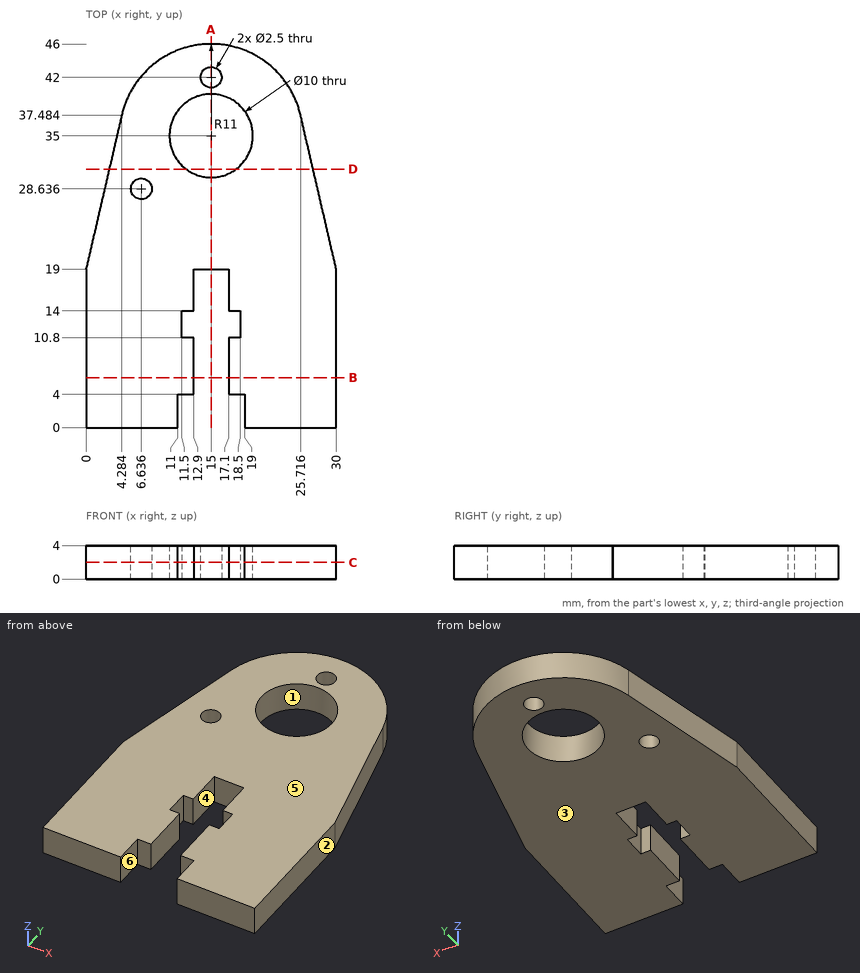
Geometry: see drawing. Coordinates: mm, zero at the bounding-box minimum. A direction names the side the tool comes from. Give positions to 0.01 mm unless a question says otherwise; leave off trailing zeros. Order: outer loops, then holes, each group sorted by start corner. A loop starts at its lowest first (then second) coordinate and runs counter-clockwise, first axis right, second up.
1. Cut plane A-A (x = 15). Return loops of the section in (y, z), and give its area (3 significant figures).
Computed:
outline: (19, 0) - (30, 0) - (30, 4) - (19, 4) - close; (40, 0) - (40.75, 0) - (40.75, 4) - (40, 4) - close; (43.25, 0) - (46, 0) - (46, 4) - (43.25, 4) - close
area: 58.0 mm2
2. Set-up query: the marked faces 5 and 6. Return all of +Z, -Z, +X, -X, +Y, -Y with unobstructed straight access to the full face (end or side cutting, diameter ignored); none if empty.
Computed:
face 5: +Z, +X, -X, +Y, -Y
face 6: +Z, -Z, -Y
3. Pin query (flat end, axial travel): pin 1 Ø1.2 at (x, z) = (15, 2.5) entering from -Y; pin 2 Ø0.7 at (x, z) = (12.5, 1.5) entering from -Y; pin 3 Ø1.1 at (x, z) = (12.5, 3) entering from +Y; pin 4 Ø2 at (x, y) = (15, 42) entering from -Z. Return the tip coordinate at first contact, or that it passes through.
Computed:
pin 1: stops at y = 19
pin 2: stops at y = 4
pin 3: stops at y = 45.83
pin 4: passes through
4. Cut plane B-B (y = 6). Return loops of the section in (x, z).
Computed:
outline: (0, 0) - (12.9, 0) - (12.9, 4) - (0, 4) - close; (17.1, 0) - (30, 0) - (30, 4) - (17.1, 4) - close
5. Cut plane C-C (z = 2). Return loops of the section in (x, y), and give its area (3 significant figures).
Computed:
outline: (0, 0) - (11, 0) - (11, 4) - (12.9, 4) - (12.9, 10.8) - (11.5, 10.8) - (11.5, 14) - (12.9, 14) - (12.9, 19) - (17.1, 19) - (17.1, 14) - (18.5, 14) - (18.5, 10.8) - (17.1, 10.8) - (17.1, 4) - (19, 4) - (19, 0) - (30, 0) - (30, 19) - (25.72, 37.48) arc R11 ccw to (4.28, 37.48) - (0, 19) - close; hole circle Ø2.5 at (6.64, 28.64); hole circle Ø10 at (15, 35); hole circle Ø2.5 at (15, 42)
area: 989 mm2
6. Draft query along X for the marked faces 1, 2, 3 and 4. Return one class per face: released by +X, released by -X, zero draft, split by the parting line, or undercut.
Computed:
face 1: undercut
face 2: released by +X
face 3: zero draft
face 4: undercut
7. Cut plane D-D (y = 31). Return loops of the section in (x, z).
Computed:
outline: (2.78, 0) - (12, 0) - (12, 4) - (2.78, 4) - close; (18, 0) - (27.22, 0) - (27.22, 4) - (18, 4) - close
8. Line query: probe 1 along Y at (x, z) = (15, 2.65); probe 2 along Y at (x, z) = (18.25, 3.7); probe 3 along X at (y, z) = (3, 3.7). Output: solid intervals per line, ascending.
Computed:
probe 1: y = 19 to 30, 40 to 40.75, 43.25 to 46
probe 2: y = 4 to 10.8, 14 to 31.2, 38.8 to 45.51
probe 3: x = 0 to 11, 19 to 30
